```python
from build123d import *

# Parameters (mm, degrees)
EXTRUDE_1_DEPTH     = 2
SKETCH_2_R          = 0.6
CUT_EXTRUDE_1_DEPTH = 18.8325545
FILLET_1_R          = 1
SKETCH_3_W          = 8
SKETCH_3_H          = 0.367219666
CUT_EXTRUDE_2_DEPTH = 18.8325545
SKETCH_4_R          = 0.55
CUT_EXTRUDE_3_DEPTH = 18.8325545


with BuildPart() as part:
    # 草图1 → 凸台-拉伸1 (new body)
    with BuildSketch(Plane(origin=(0, 0, 0), x_dir=(1, 0, 0), z_dir=(0, 1, 0))):
        Polygon((17, 2), (14, 5), (0, 5), (0, 0), (17, 0), align=None)
    extrude(amount=EXTRUDE_1_DEPTH)

    # 草图2 → 切除-拉伸1 (cut, through all)
    with BuildSketch(Plane(origin=(17, 0, 0), x_dir=(0, 0, -1), z_dir=(1, 0, 0))):
        with Locations((1, 1)):
            Circle(SKETCH_2_R)
    extrude(amount=-CUT_EXTRUDE_1_DEPTH, mode=Mode.SUBTRACT)

    # 圆角1
    fillet_1_edges = [part.edges().sort_by_distance(p)[0] for p in [
        (7, 0, -5),
        (7, 2, -5),
    ]]
    fillet(fillet_1_edges, radius=FILLET_1_R - 0.0001)  # a hair under: the kernel refuses the full size

    # 草图3 → 切除-拉伸2 (cut, through all)
    with BuildSketch(Plane.ZY):
        with Locations((0, 1)):
            Rectangle(SKETCH_3_W, SKETCH_3_H)
    extrude(amount=-CUT_EXTRUDE_2_DEPTH, mode=Mode.SUBTRACT)

    # 草图4 → 切除-拉伸3 (cut, through all)
    with BuildSketch(Plane(origin=(0, 2, 0), x_dir=(1, 0, 0), z_dir=(0, 1, 0))):
        with Locations(Location((10, 2, 0), (0, 0, 270))):
            Circle(SKETCH_4_R)
    extrude(amount=-CUT_EXTRUDE_3_DEPTH, mode=Mode.SUBTRACT)


solid = part.part
```
Verification items for the finished model (mm, model axes). A direction names the side the tool comes from. Give positions to 0.01 mm unless a question says otherwise; leave off trailing zeros. Order: outer loops, then holes, each group sorted by start corner. A loop starts at its lowest first (then second) coordinate and runs counter-clockwise, first axis right, second up. Notation, with made-up numbers: M 58,52.5 L 76,52.5 A29 ccw 76,79.5 Z; hole C -9.5,87.25 d6. An arc over 180 degrees is marked long. Return JSON: item names as keys, results as strings. Group by question number.
1) Section check D-D on y = 0.25. Record the cut outline in (x, z).
2) Section check A-A on z = -2.75. Record the cut outline in (x, y).
3) Scan lines: line 1 (Y direction, x = 8.5, z = -2.3); line 2 (Z direction, x = 10.25, y = 0.5); line 3 (X direction, y = 0.7, z = -1.9). Record each from-to range of solid material in increasing order.
4) Section check B-B on x = 10. Give the number of separate pieces and of enclosed holes in the cut face, and give its area (3 significant figures).
5) Mould release check, pull along Y, two halves, no side actions. Record for faces 4 (the face through (8, 1.184, -3)), 5 (the face through (15.5, 1.4, -3.5)), 6 (the face through (8, 0, -2)): pulls with the +Y half, pulls with the -Y half, needs draft (parallel to the pull), parting line crosses it, or undercut.
6) Access from +Z, -Z, +X, -X, +Y, -Y to the whole of each face (thin tool, end or side, straight path). Record for faces 1 (the face through (10.02, 0.41, -2.55)), 2 (the face through (8, 0.816, -3)), 3 (the face through (8.6, 1.6, -1)).
Answer block:
{
 "1": {"outline": "M 0,-4.66 L 14.34,-4.66 L 17,-2 L 17,0 L 0,0 Z; hole C 10,-2 d1.1"},
 "2": {"outline": "M 0,0 L 16.25,0 L 16.25,0.82 L 0,0.82 Z; M 0,1.18 L 16.25,1.18 L 16.25,2 L 0,2 Z"},
 "3": {"line 1": "y = 0 to 0.82, 1.18 to 2", "line 2": "z = -4.87 to -2.49, -1.51 to -1.33, -0.67 to 0", "line 3": "x = 0 to 9.46, 10.54 to 17"},
 "4": {"separate pieces": "3", "enclosed holes": "0", "area": "5.64 mm^2"},
 "5": {"face 4": "undercut", "face 5": "needs draft", "face 6": "pulls with the -Y half"},
 "6": {"face 1": "+Y, -Y", "face 2": "+Z, +X, -X", "face 3": "+X, -X"}
}
